Part model, mm, in its own coordinate system. Face numbers are marked on the shaded views. A direction names the side the tool comes from. Round coordinates to 2 decimals unless told otherwise and drop trailing zeros. Order: outer loops, then holes, each group sorted by start corner. A loop starts at its lowest first (then second) coordinate and runs counter-clockwise, first axis right, second up. Notation, with made-up numbers: (-10.75, 45.5) - (11.25, 45.5) arc R30 ccw to (11.25, 79.5) - close; hole circle Ø6 at (30.5, 57). An arc over 180 degrees is marked (long way). Answer as a JSON object with one key per item and string values.
```python
from build123d import *

# Parameters (mm, degrees)
EXTRUDE_1_DEPTH     = 60
SKETCH_2_R          = 12.5
CUT_EXTRUDE_1_DEPTH = 81


with BuildPart() as part:
    # Эскиз1 → Бобышка-Вытянуть1 (new body)
    with BuildSketch(Plane(origin=(0, 0, 0), x_dir=(1, 0, 0), z_dir=(0, 1, 0))):
        with BuildLine():
            Line((0, 80), (0, 5))
            ThreePointArc((0, 5), (1.464466094, 1.464466094), (5, 0))
            Line((5, 0), (53, 0))
            ThreePointArc((53, 0), (56.535533906, 1.464466094), (58, 5))
            Line((58, 5), (58, 80))
            Line((58, 80), (53, 80))
            Line((53, 80), (53, 10.822157735))
            ThreePointArc((53, 10.822157735), (51.535533906, 7.286623829), (48, 5.822157735))
            Line((48, 5.822157735), (10, 5.822157735))
            ThreePointArc((10, 5.822157735), (6.464466094, 7.286623829), (5, 10.822157735))
            Line((5, 10.822157735), (5, 80))
            Line((5, 80), (0, 80))
        make_face()
    extrude(amount=EXTRUDE_1_DEPTH)

    # Эскиз2 → Вырез-Вытянуть1 (cut, through all)
    with BuildSketch(Plane.XY):
        with Locations((29, 30)):
            Circle(SKETCH_2_R)
    extrude(amount=-CUT_EXTRUDE_1_DEPTH, mode=Mode.SUBTRACT)


solid = part.part
```
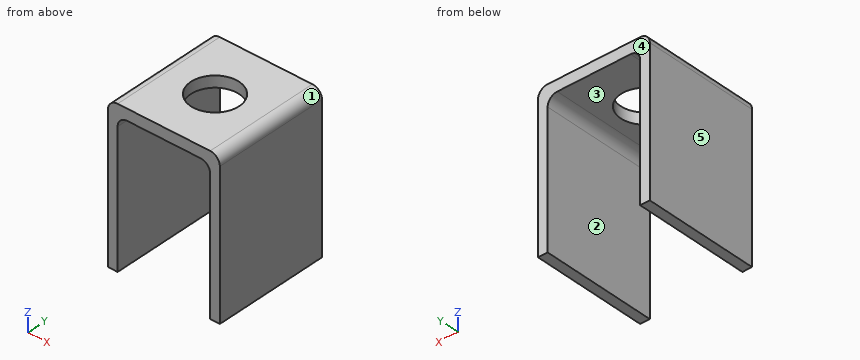
Item 1: Cut at A-A (y = 30). Write the cut outline in (x, z), plus the area to 3 significant figures.
Taken from the geometry:
{"outline": "(0, -80) - (5, -80) - (5, -10.82) arc R5 cw to (10, -5.82) - (16.5, -5.82) - (16.5, 0) - (5, 0) arc R5 ccw to (0, -5) - close; (41.5, -5.82) - (48, -5.82) arc R5 cw to (53, -10.82) - (53, -80) - (58, -80) - (58, -5) arc R5 ccw to (53, 0) - (41.5, 0) - close", "area": "934 mm2"}
Item 2: Drop a flat-ended pin along its axis: P1, Ø19, axis at x = 20, y = 18, coming from the -Z side. Give the stop position or say it passes through.
Taken from the geometry:
{"P1": "z = -5.82"}
Item 3: Cut at C-C (z = -21). Write the cut outline in (x, y), plus the area to 3 significant figures.
Taken from the geometry:
{"outline": "(0, 0) - (5, 0) - (5, 60) - (0, 60) - close; (53, 0) - (58, 0) - (58, 60) - (53, 60) - close", "area": "600 mm2"}
Item 4: Cut at B-B (x = 29). Write the cut outline in (y, z).
Taken from the geometry:
{"outline": "(0, -5.82) - (17.5, -5.82) - (17.5, 0) - (0, 0) - close; (42.5, -5.82) - (60, -5.82) - (60, 0) - (42.5, 0) - close"}
Item 5: Probe L1, parallel to Y at x = 29, z = -2.1; L2, parallel to X at y = 37, z = -23; L3, parallel to Z at x = 31, y = 11.5. List the from-to ranges inside material, lowest first. Write a range as from..to.
Taken from the geometry:
{"L1": "0..17.5, 42.5..60", "L2": "0..5, 53..58", "L3": "-5.82..0"}
Item 6: Two-plate mould, pull along X, no slides. Class the marked faces 3, 4 and 5: pulls with the +X half, pulls with the -X half, needs draft (parallel to the pull), parting line crosses it, or undercut.
Taken from the geometry:
{"face 3": "undercut", "face 4": "needs draft", "face 5": "pulls with the -X half"}
Item 7: Tool access for the marked faces 1 and 2: list every direction of +Z, -Z, +X, -X, +Y, -Y with a clear straight run to the whole face (end or side of a thin tool).
Taken from the geometry:
{"face 1": "+Z, +X, +Y, -Y", "face 2": "-Z, +Y, -Y"}
Item 8: Cut at D-D (y = 14). Write the cut outline in (x, z).
Taken from the geometry:
{"outline": "(0, -80) - (5, -80) - (5, -10.82) arc R5 cw to (10, -5.82) - (48, -5.82) arc R5 cw to (53, -10.82) - (53, -80) - (58, -80) - (58, -5) arc R5 ccw to (53, 0) - (5, 0) arc R5 ccw to (0, -5) - close"}
